For this review, take the finished solid that the model builds, in its own axes (mm). A direction names the side the tool comes from. Round coordinates to 2 decimals unless told otherwise and drop trailing zeros. Loops run counter-clockwise (first coordinate to the right, second up) from the corner with the lowest first, then second, coordinate; pieces in that order, holes last.
1. To check wall thickness, follow line 1 along Z through (x, y) = (4, 0); line 2 along X through (y, z) = (6.25, -0.5); line 3 along Y through (x, z) = (22.5, -0.5). State the ranges of each line that lie inside material, in increasing order.
2. Clearance check with flat-ended pins moving along their axes: pin 1 Ø5 at (x, y) = (160, -6) entering from -Z; pin 2 Ø3.5 at (y, z) = (-2, -1.5) entering from -X; pin 3 Ø1.2 at (x, y) = (28, -0.5) entering from +Z; pin 4 Ø3 at (x, z) = (120, 1) entering from -Y. State where each tip first meets the part, or that it passes through.
3. Consider section B-B on x = 157.5. State the section outline as (y, z) points, then the cut area to 3 significant figures.
4. Consider section A-A on x = 17. State the section outline as (y, z) points, then the cut area to 3 significant figures.
5. Draft analysis for pull direction X (two halves, no side actions). For faces 1 (the flat face through (169, -6, -2)), 2 (the flat face through (150, -2, 7)), 3 (the flat face through (132, -6, 2)), state which applies: released by +X, released by -X, zero draft, split by the parting line, or undercut.
6. Consider section C-C on x = 64. State the section outline as (y, z) points.
7. Tool access review of faces 4 (the cylindrical face through (134.942, 7.907, -1.756)), 5 (the cylindrical face through (173, 0, -6)), 6 (the flat face through (182, 0, 0)), 7 (the cylindrical face through (150.29, -7.167, 4.57)), 8 (the flat face through (7, 0, 0)): name each direction out of +Z, -Z, +X, -X, +Y, -Y from which nothing blocks a thin tool from reaching the whole face with its end or side.
from build123d import *

# Parameters (mm, degrees)
F4_DEPTH = 3
F7_DEPTH = 3
F8_R     = 2.1
F9_DEPTH = 7
F10_SIZE = 0.5


with BuildPart() as f1:
    # F0 (on Front) → F1 (revolve)
    with BuildSketch(Plane.XZ):
        Polygon((0, 5.5), (0, 0), (182, 0), (182, 6), (178.6, 6), (178.6, 5.75), (177.5, 5.75), (177.5, 6), (169, 6), (169, 8.5), (166.6, 8.5), (166.6, 8.1), (165.5, 8.1), (165.5, 8.5), (135.5, 8.5), (135.5, 8.1), (134.4, 8.1), (134.4, 8.5), (132, 8.5), (132, 6), (125.5, 6), (125.5, 5.75), (124.4, 5.75), (124.4, 6), (121, 6), (121, 5.5), align=None)
    revolve(axis=Axis((91, 0, 0), (1, 0, 0)))

    # F3 (on offset) → F4 (cut)
    with BuildSketch(Plane.XY.offset(5.5)):
        with BuildLine():
            Line((0, 2), (0, -2))
            Line((0, -2), (44, -2))
            ThreePointArc((44, -2), (45.414214, -1.414214), (46, 0))
            ThreePointArc((46, 0), (45.414214, 1.414214), (44, 2))
            Line((44, 2), (0, 2))
        make_face()
    extrude(amount=-F4_DEPTH, mode=Mode.SUBTRACT)

    # F6 (on offset) → F7 (cut)
    with BuildSketch(Plane.XY.offset(8.5)):
        with BuildLine():
            ThreePointArc((138, 0.5), (138.732233, -1.267767), (140.5, -2))
            Line((140.5, -2), (160.5, -2))
            ThreePointArc((160.5, -2), (162.267767, -1.267767), (163, 0.5))
            ThreePointArc((163, 0.5), (162.267767, 2.267767), (160.5, 3))
            Line((160.5, 3), (140.5, 3))
            ThreePointArc((140.5, 3), (138.732233, 2.267767), (138, 0.5))
        make_face()
    extrude(amount=-F7_DEPTH, mode=Mode.SUBTRACT)

    # F8 (on face) → F9 (cut)
    with BuildSketch(Plane(origin=(0, 0, 0), x_dir=(0, -1, 0), z_dir=(-1, 0, 0))):
        Circle(F8_R)
    extrude(amount=-F9_DEPTH, mode=Mode.SUBTRACT)

    # F10
    f10_edges = [f1.edges().sort_by_distance(p)[0] for p in [
        (182, 0, -6),
    ]]
    chamfer(f10_edges, length=F10_SIZE)


solid = f1.part
Resolved:
1. line 1: z = -5.5 to -2.1, 2.1 to 2.5
1. line 2: x = 132 to 169
1. line 3: y = -5.48 to 5.48
2. pin 1: stops at z = -7.75
2. pin 2: stops at x = 0
2. pin 3: stops at z = 2.5
2. pin 4: stops at y = -6
3. outline: (-2, 5.5) - (-2, 8.26) arc R8.5 ccw (long way) to (3, 7.95) - (3, 5.5) - close
3. area: 213 mm2
4. outline: (-2, 2.5) - (-2, 5.12) arc R5.5 ccw (long way) to (2, 5.12) - (2, 2.5) - close
4. area: 83.5 mm2
5. face 1: released by +X
5. face 2: undercut
5. face 3: released by -X
6. outline: circle Ø11 at (0, 0)
7. face 4: none
7. face 5: +X
7. face 6: +Z, -Z, +X, +Y, -Y
7. face 7: +X, -X
7. face 8: -X
